Can you work these out from the model? Positions are in its coordinate system, mm. Face numbers are marked on the shaded views. Round coordinates to 2 decimals unless told otherwise and drop trailing zeros. Loops run counter-clockwise (first coordinate to the right, second up) from the corner with the lowest first, then second, coordinate; pieces in that order, holes last.
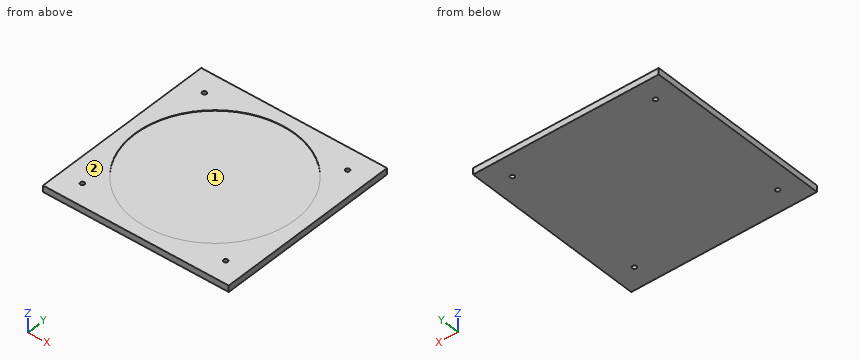
from build123d import *

# Parameters (mm, degrees)
F0_W     = 175
F0_H     = 175
F1_DEPTH = 6
F2_R     = 75.5
F3_DEPTH = 0.5
F4_R     = 2
F5_DEPTH = 6.001


with BuildPart() as f1:
    # F0 (on Top) → F1 (new body)
    with BuildSketch(Plane.XY):
        with Locations((87.5, 87.5)):
            Rectangle(F0_W, F0_H)
    extrude(amount=F1_DEPTH)

    # F2 (on face) → F3 (cut)
    with BuildSketch(Plane.XY.offset(6)):
        with Locations((87.5, 87.5)):
            Circle(F2_R)
    extrude(amount=-F3_DEPTH, mode=Mode.SUBTRACT)

    # F4 (on face) → F5 (cut, through all)
    with BuildSketch(Plane.XY.offset(6)):
        with Locations((20, 155)):
            Circle(F4_R)
        with Locations((155, 155)):
            Circle(F4_R)
        with Locations((155, 20)):
            Circle(F4_R)
        with Locations((20, 20)):
            Circle(F4_R)
    extrude(amount=-F5_DEPTH, mode=Mode.SUBTRACT)


solid = f1.part
(1) If I drill on line 1 (X direction, y = 155, z = 4.1); line 2 (Z direction, x = 40, y = 68), over which ranges is the centre line in solid material (lowest first)?
Worked answers:
line 1: x = 0 to 18, 22 to 153, 157 to 175
line 2: z = 0 to 5.5
(2) Will these pins go through, and if not, where does the flat tip stop? P1, Ø3.5, axis at x = 20, y = 155, coming from the -Z side; P2, Ø3, axis at x = 33, y = 23.5, coming from the -Z side.
Worked answers:
P1: passes through
P2: stops at z = 0
(3) If we mould it in two halves opening along X, with no side actions, what happens to the marked faces 1 and 2? For each: released by +X, released by -X, zero draft, split by the parting line, or undercut.
Worked answers:
face 1: undercut
face 2: zero draft
(4) If we section it at A-A, the plane y = 87.5: List the corners of the cut face in (x, z) for me.
Worked answers:
outline: (0, 0) - (175, 0) - (175, 6) - (163, 6) - (163, 5.5) - (12, 5.5) - (12, 6) - (0, 6) - close
(5) If we section it at B-B, the plane y = 155: List the corners of the cut face in (x, z) for me, then the cut area to 3 significant figures.
Worked answers:
outline: (0, 0) - (18, 0) - (18, 6) - (0, 6) - close; (22, 0) - (153, 0) - (153, 6) - (121.32, 6) - (121.32, 5.5) - (53.68, 5.5) - (53.68, 6) - (22, 6) - close; (157, 0) - (175, 0) - (175, 6) - (157, 6) - close
area: 968 mm2
